Source: CAD feature listing. Evaluate the final solid. Frame: model axes, mm. Round coordinates to 2 decimals unless told otherwise and drop trailing zeros.
Autodesk Inventor part; units mm, degrees
ref_plane "YZ Plane" through (0, 0, 0) normal (1, 0, 0) x (0, 1, 0)
ref_plane "XZ Plane" through (0, 0, 0) normal (0, 1, 0) x (-1, 0, 0)
ref_plane "XY Plane" through (0, 0, 0) normal (0, 0, 1) x (1, 0, 0)
sketch "Náčrt1" plane through (0, 0, 0) normal (0, 0, 1) x (1, 0, 0)
  line L0 (-7.5, -1) -> (7.5, -1)
  line L1 (7.5, -1) -> (7.5, 1)
  line L2 (7.5, 1) -> (-7.5, 1)
  line L3 (-7.5, 1) -> (-7.5, -1)
  line L4 (-7.5, -1) -> (7.5, 1) construction
  line L5 (7.5, -1) -> (-7.5, 1) construction
  point P0 (0, 0)
  dimension "d0" = 15
  dimension "d1" = 2
extrude "Vysunutí1" add sketch "Náčrt1" along normal blind 640
sketch "Náčrt2" plane through (-7.5, 1, 0) normal (0, 1, 0) x (1, 0, 0)
  line L0 (15, 0) -> (0, 0)
  line L1 (0, 0) -> (0, -640)
  line L2 (15, -640) -> (0, -640)
  line L3 (15, 0) -> (15, -640)
  circle A0 centre (7.5, -7.5) radius 1.5
  line L4 (15, 0) -> (15, -640)
  line L5 (15, -320) -> (0, -320)
  circle A1 centre (7.5, -632.5) radius 1.5
  point P0 (7.5, 0)
  dimension "d4" = 7.5
  dimension "d6" = 7.5
  dimension "d7" = 3
extrude "Vysunutí2" cut sketch "Náčrt2" against normal up to next contours A0 | A1
sketch "Náčrt3" plane through (-7.5, 1, 0) normal (0, 1, 0) x (1, 0, 0)
  line L0 (15, 0) -> (15, -640)
  line L1 (0, 0) -> (0, -640)
  circle A0 centre (7.5, -320) radius 1.5
  line L2 (15, 0) -> (0, 0)
  point P0 (7.5, 0)
  dimension "d11" = 3
  dimension "d12" = 7.5
  dimension "d13" = 320
extrude "Vysunutí3" cut sketch "Náčrt3" against normal up to next
pattern_linear "Obdélníkové pole1" count 12 spacing 25.4 along (0, 0, 1) count 12 spacing 25.4 along (0, 0, -1) of "Vysunutí3"
equation "\"d0\" = width"
equation "\"d1\" = thickness"
equation "\"d2\" = length"
equation "\"d4\" = 0.5 * width"
equation "\"d6\" = 0.5 * width"
equation "\"d7\" = holeDia"
equation "\"d8\" = length"
equation "\"d12\" = 0.5 * width"
equation "\"d13\" = 0.5 * length"
equation "\"d14\" = length"
equation "\"d16\" = 0.5 * holeCount"
equation "\"d18\" = holeDistance"
equation "\"d19\" = 0.5 * holeCount"
equation "\"d21\" = holeDistance"
equation "\"length\" = gCabinet_FerriteCore_Width"
equation "\"width\" = 15"
equation "\"thickness\" = 2"
equation "\"holeDia\" = 3"
equation "\"holeDistance\" = 25.4"
properties part number "Profile-Flat-01"
1) Material intervals for line 1 (X direction, y = 0.45, z = 167.6), sorted ascending.
Taken from the geometry:
line 1: x = -7.5 to -1.5, 1.5 to 7.5
2) Contact query for a flat-ended pin moving along its axis: P1, Ø2.5, axis at x = 0, z = 116.8, coming from the -Y side. Output: stop coordinate, or through.
Taken from the geometry:
P1: passes through
3) Section query A-A on y = 0. State how many separate pieces and enclosed holes the cut face has, then the cut area to 3 significant figures.
Taken from the geometry:
separate pieces: 1
enclosed holes: 25
area: 9,420 mm2
